Verification items for the finished model (mm, model axes). A direction names the side the tool comes from. Give positions to 0.01 mm unless a question says otherwise; leave off trailing zeros. Write each loop counter-clockwise with the first axis right and the second up, starting at its lowest first coordinate (ties: lowest second). Pieces come first, ordered by that corner, then holes.
from build123d import *

# Parameters (mm, degrees)
F2_DEPTH       = 2
F3_W           = 13.9999988079
F3_H           = 18
F4_DEPTH       = 2.001
F6_DEPTH       = 6
F7_R           = 1.8
F8_DEPTH       = 6.001
F10_R          = 3.4
F11_DEPTH      = 1.4
F11_DEPTH_BACK = 1.4
F13_W          = 6.8
F13_H          = 2.8
F14_DEPTH      = 8.8
F16_W          = 6.8
F16_H          = 2.8
F17_DEPTH      = 10.3
F18_W          = 8
F18_H          = 2
F19_DEPTH      = 16
F21_DEPTH      = 2.001


# Not quite as in the source:
# - after a boolean that leaves OpenCascade's solid faulty, fix() repairs it
# - a feature names something its author has since deleted; it is built from what else it names


with BuildPart() as f2:
    # F1 (on Top) → F2 (new body)
    with BuildSketch(Plane.XY):
        Polygon((29, 29), (29, 37.5), (-29, 37.5), (-29, 29), (-37.5, 29), (-37.5, -29), (-29, -29), (-29, -37.5), (29, -37.5), (29, -29), (37.5, -29), (37.5, 29), align=None)
    extrude(amount=F2_DEPTH)

    # F3 (on face) → F4 (cut, through all)
    with BuildSketch(Plane.XY.offset(2)):
        with Locations((-25.499999404, 12)):
            Rectangle(F3_W, F3_H)
        with Locations((-25.499999404, -12)):
            Rectangle(F3_W, F3_H)
        Polygon((-12.5, -32.5), (21, -32.5), (21, -21), (30.5, -21), (30.5, 21), (21, 21), (21, 32.5), (-12.5, 32.5), align=None)
    extrude(amount=-F4_DEPTH, mode=Mode.SUBTRACT)

    # F5 (on face) → F6 (join)
    with BuildSketch(Plane.XY.offset(2)):
        with BuildLine():
            ThreePointArc((-23.4949874371, 21), (-23.3511822993, 24.0860292221), (-20.7, 22.5))
            ThreePointArc((-20.7, 22.5), (-20.9139707779, 21.6488177007), (-21.5050125629, 21))
            Line((-21.5050125629, 21), (-18.5, 21))
            Line((-18.5, 21), (-18.5, 18.7250827824))
            ThreePointArc((-18.5, 18.7250827824), (-17.3887379249, 20.4689903988), (-17, 22.5))
            ThreePointArc((-17, 22.5), (-23.2572105316, 27.9476262914), (-27.7915026221, 21))
            Line((-27.7915026221, 21), (-23.4949874371, 21))
        make_face()
        with BuildLine():
            ThreePointArc((-21.5050125629, 21), (-22.5, 20.7), (-23.4949874371, 21))
            Line((-23.4949874371, 21), (-27.7915026221, 21))
            ThreePointArc((-27.7915026221, 21), (-23.8079781506, 17.1577913596), (-18.5, 18.7250827824))
            Line((-18.5, 18.7250827824), (-18.5, 21))
            Line((-18.5, 21), (-21.5050125629, 21))
        make_face()
        with BuildLine():
            ThreePointArc((-21.5050125629, -21), (-20.9139707779, -21.6488177007), (-20.7, -22.5))
            ThreePointArc((-20.7, -22.5), (-23.3511822993, -24.0860292221), (-23.4949874371, -21))
            Line((-23.4949874371, -21), (-27.7915026221, -21))
            ThreePointArc((-27.7915026221, -21), (-23.2572105316, -27.9476262914), (-17, -22.5))
            ThreePointArc((-17, -22.5), (-17.3887379249, -20.4689903988), (-18.5, -18.7250827824))
            Line((-18.5, -18.7250827824), (-18.5, -21))
            Line((-18.5, -21), (-21.5050125629, -21))
        make_face()
        with BuildLine():
            ThreePointArc((-23.4949874371, -21), (-22.5, -20.7), (-21.5050125629, -21))
            Line((-21.5050125629, -21), (-18.5, -21))
            Line((-18.5, -21), (-18.5, -18.7250827824))
            ThreePointArc((-18.5, -18.7250827824), (-23.8079781506, -17.1577913596), (-27.7915026221, -21))
            Line((-27.7915026221, -21), (-23.4949874371, -21))
        make_face()
        with BuildLine():
            ThreePointArc((21, 23.4949874371), (23.0196152423, 24.223368794), (24.3, 22.5))
            ThreePointArc((24.3, 22.5), (24.0860292221, 21.6488177007), (23.4949874371, 21))
            Line((23.4949874371, 21), (27.7915026221, 21))
            ThreePointArc((27.7915026221, 21), (27.9476262914, 21.7427894684), (28, 22.5))
            ThreePointArc((28, 22.5), (25.8166247904, 26.8874821937), (21, 27.7915026221))
            Line((21, 27.7915026221), (21, 23.4949874371))
        make_face()
        with BuildLine():
            ThreePointArc((21, 21.5050125629), (20.7, 22.5), (21, 23.4949874371))
            Line((21, 23.4949874371), (21, 27.7915026221))
            ThreePointArc((21, 27.7915026221), (18.6109127035, 18.6109127035), (27.7915026221, 21))
            Line((27.7915026221, 21), (23.4949874371, 21))
            ThreePointArc((23.4949874371, 21), (22.5, 20.7), (21.5050125629, 21))
            Line((21.5050125629, 21), (21, 21))
            Line((21, 21), (21, 21.5050125629))
        make_face()
        with BuildLine():
            ThreePointArc((21.5050125629, 21), (21.2272077939, 21.2272077939), (21, 21.5050125629))
            Line((21, 21.5050125629), (21, 21))
            Line((21, 21), (21.5050125629, 21))
        make_face()
        with BuildLine():
            Line((23.4949874371, -21), (27.7915026221, -21))
            ThreePointArc((27.7915026221, -21), (18.6109127035, -18.6109127035), (21, -27.7915026221))
            Line((21, -27.7915026221), (21, -23.4949874371))
            ThreePointArc((21, -23.4949874371), (20.7, -22.5), (21, -21.5050125629))
            Line((21, -21.5050125629), (21, -21))
            Line((21, -21), (21.5050125629, -21))
            ThreePointArc((21.5050125629, -21), (22.5, -20.7), (23.4949874371, -21))
        make_face()
        with BuildLine():
            ThreePointArc((28, -22.5), (27.9476262914, -21.7427894684), (27.7915026221, -21))
            Line((27.7915026221, -21), (23.4949874371, -21))
            ThreePointArc((23.4949874371, -21), (24.0860292221, -21.6488177007), (24.3, -22.5))
            ThreePointArc((24.3, -22.5), (23.0196152423, -24.223368794), (21, -23.4949874371))
            Line((21, -23.4949874371), (21, -27.7915026221))
            ThreePointArc((21, -27.7915026221), (25.8166247904, -26.8874821937), (28, -22.5))
        make_face()
        with BuildLine():
            ThreePointArc((21, -21.5050125629), (21.2272077939, -21.2272077939), (21.5050125629, -21))
            Line((21.5050125629, -21), (21, -21))
            Line((21, -21), (21, -21.5050125629))
        make_face()
    extrude(amount=-F6_DEPTH)

    # F7 (on face) → F8 (cut, through all)
    with BuildSketch(Plane(origin=(0, 0, -4), x_dir=(1, 0, 0), z_dir=(0, 0, -1))):
        with Locations((-22.5, -22.5)):
            Circle(F7_R)
        with Locations((-22.5, 22.5)):
            Circle(F7_R)
        with Locations((22.5, -22.5)):
            Circle(F7_R)
        with Locations((22.5, 22.5)):
            Circle(F7_R)
    extrude(amount=-F8_DEPTH, mode=Mode.SUBTRACT)

    add(f2.part.fix(), mode=Mode.REPLACE)

    # F10 (on offset) → F11 (cut, two sides)
    with BuildSketch(Plane.XY.offset(-1)) as f11_sk:
        with Locations((22.5, -22.5)):
            Circle(F10_R)
        with Locations((22.5, 22.5)):
            Circle(F10_R)
        with Locations((-22.5, -22.5)):
            Circle(F10_R)
        with Locations((-22.5, 22.5)):
            Circle(F10_R)
    extrude(amount=-F11_DEPTH, mode=Mode.SUBTRACT)
    extrude(f11_sk.sketch, amount=F11_DEPTH_BACK, mode=Mode.SUBTRACT)

    # F13 (on offset) → F14 (cut)
    with BuildSketch(Plane.XZ.offset(22.5)):
        with Locations((22.5, -1)):
            Rectangle(F13_W, F13_H)
        with Locations((-22.5, -1)):
            Rectangle(F13_W, F13_H)
    extrude(amount=-F14_DEPTH, mode=Mode.SUBTRACT)

    # F16 (on offset) → F17 (cut)
    with BuildSketch(Plane.XZ.offset(-22.5)):
        with Locations((22.5, -1)):
            Rectangle(F16_W, F16_H)
        with Locations((-22.5, -1)):
            Rectangle(F16_W, F16_H)
    extrude(amount=F17_DEPTH, mode=Mode.SUBTRACT)

    # F18 (on face) → F19 (join)
    with BuildSketch(Plane(origin=(30.5, 0, 0), x_dir=(0, -1, 0), z_dir=(-1, 0, 0))):
        with Locations((0, 1)):
            Rectangle(F18_W, F18_H)
    extrude(amount=F19_DEPTH)

    # F20 (on face) → F21 (cut, through all)
    with BuildSketch(Plane(origin=(0, 0, 0), x_dir=(1, 0, 0), z_dir=(0, 0, -1))):
        with BuildLine():
            ThreePointArc((-25, 30.6240384046), (-19.7091840098, 30.5287823553), (-15.4999997467, 27.3218250127))
            Line((-15.4999997467, 27.3218250127), (-15.4999997467, 33.5))
            Line((-15.4999997467, 33.5), (-25, 33.5))
            Line((-25, 33.5), (-25, 30.6240384046))
        make_face()
        with BuildLine():
            Line((-25, -33.5), (-15.4999997467, -33.5))
            Line((-15.4999997467, -33.5), (-15.4999997467, -27.3218250127))
            ThreePointArc((-15.4999997467, -27.3218250127), (-19.7091840098, -30.5287823553), (-25, -30.6240384046))
            Line((-25, -30.6240384046), (-25, -33.5))
        make_face()
    extrude(amount=-F21_DEPTH, mode=Mode.SUBTRACT)


solid = f2.part
Item 1: Sectioned sample at B-B on y = 11. Record the cut outline in (x, z).
Answer key:
outline: (-37.5, 0) - (-32.5, 0) - (-32.5, 2) - (-37.5, 2) - close; (-18.5, 0) - (-12.5, 0) - (-12.5, 2) - (-18.5, 2) - close; (30.5, 0) - (37.5, 0) - (37.5, 2) - (30.5, 2) - close
Item 2: Set-up check for faces 1 (the face through (21, 30, 1)), 2 (the face through (25.9, -20, -1)), 3 (the face through (0, 37.5, 1)): record each of +Z, -Z, +X, -X, +Y, -Y from which the full face is reachable in a straight line by a thin tool's end or side.
Answer key:
face 1: +Z, -Z
face 2: none
face 3: +Z, -Z, +X, -X, +Y
Item 3: Release check for a two-part mould opening along X. For faces 4 (the face through (37.5, 0, 1)), 5 (the face through (-32.5, 12, 1)), 6 (the face through (-33, 29, 1)) record: released by +X, released by -X, zero draft, split by the parting line, or undercut.
Answer key:
face 4: released by +X
face 5: undercut
face 6: zero draft
Item 4: Scan lines: line 1 along X through (y, z) = (-22.5, -3); line 2 along Y through (x, z) = (22.5, 1.3). Record each from-to range of solid material in increasing order.
Answer key:
line 1: x = -28 to -24.3, -20.7 to -17, 17 to 20.7, 24.3 to 28
line 2: y = -37.5 to -24.3, -20.7 to -17, -4 to 4, 17 to 20.7, 24.3 to 37.5
Item 5: Sectioned sample at C-C on z = -1.3. Record the cut outline in (x, y).
Answer key:
outline: (-25.9, -22.5) - (-25.9, -18.18) arc R5.5 ccw (long way) to (-19.1, -18.18) - (-19.1, -22.5) arc R3.4 cw to start; (-25.9, 18.18) - (-25.9, 22.5) arc R3.4 cw to (-19.1, 22.5) - (-19.1, 18.18) arc R5.5 ccw (long way) to start; (19.1, -22.5) - (19.1, -18.18) arc R5.5 ccw (long way) to (25.9, -18.18) - (25.9, -22.5) arc R3.4 cw to start; (19.1, 18.18) - (19.1, 22.5) arc R3.4 cw to (25.9, 22.5) - (25.9, 18.18) arc R5.5 ccw (long way) to start
Item 6: Depth check by flat-ended pin: pin 1 (0.6 mm diameter, centred on x = -30, z = 1, fed in from -Y); pin 2 (0.6 mm diameter, centred on y = -32.5, z = 1, fed in from +X); pin 3 (1.4 mm diameter, centred on y = 20.5, z = -1.5, fed in from +X). Enter the tip coordinate at first touch or a pass-through.
Answer key:
pin 1: stops at y = -29
pin 2: stops at x = 29
pin 3: stops at x = 27.84
Item 7: Sectioned sample at A-A on x = 12. Record the cut outline in (y, z), then the cut area to 3 significant figures.
Answer key:
outline: (-37.5, 0) - (-32.5, 0) - (-32.5, 2) - (-37.5, 2) - close; (32.5, 0) - (37.5, 0) - (37.5, 2) - (32.5, 2) - close
area: 20.0 mm2
Item 8: Sectioned sample at D-D on x = -22.5. State how many separate pieces and enclosed holes the cut face has, then the cut area to 3 significant figures.
Answer key:
separate pieces: 9
enclosed holes: 0
area: 99.1 mm2
